Design review of the part shown in the three views and the two pictorial views. Dimensions are in mm from the part's minimum x, y and z. Coordinates: 2 decimals unless noted, no trailing zeros. Loops run counter-clockwise (first coordinate to the right, second up) from the corner with the lowest first, then second, coordinate; pieces in that order, holes last. Notation, with made-up numbers: M 79,-28 L 98,-28 A26 cw 98,-11 Z; hole C 76,-8.5 d1. An arc over 180 degrees is marked long. Put each result on its own line as item: value. Start each with the question number.
(1) Take a section at B-B, the plane y = 2.35. Give the boundary of the cut face in (x, z), then the cut area to 3 significant figures.
(2) Take a section at A-A, the plane z = 14. Give the boundary of the cut face in (x, y), then the cut area to 3 significant figures.
(3) Clearance check with flat-ended pins moving along their axes: pin 1 (1.2 mm diameter, centred on x = 9, z = 29.5, fed in from -Y); pin 2 (3 mm diameter, centred on y = 2, z = 54, fed in from -X); pin 3 (1.2 mm diameter, centred on y = 3, z = 60.5, fed in from +X). State where each tip first meets the part, or that it passes through.
(4) For probe 1 along X at (y, z) = (3.15, 37); probe 2 along Y at (x, z) = (2.5, 58.5), list the stretches that pass through material, from the lowest coordinate up. Write a range as [from, to].
(5) Take a section at C-C, the plane x = 1.5. Give the boundary of the cut face in (y, z).
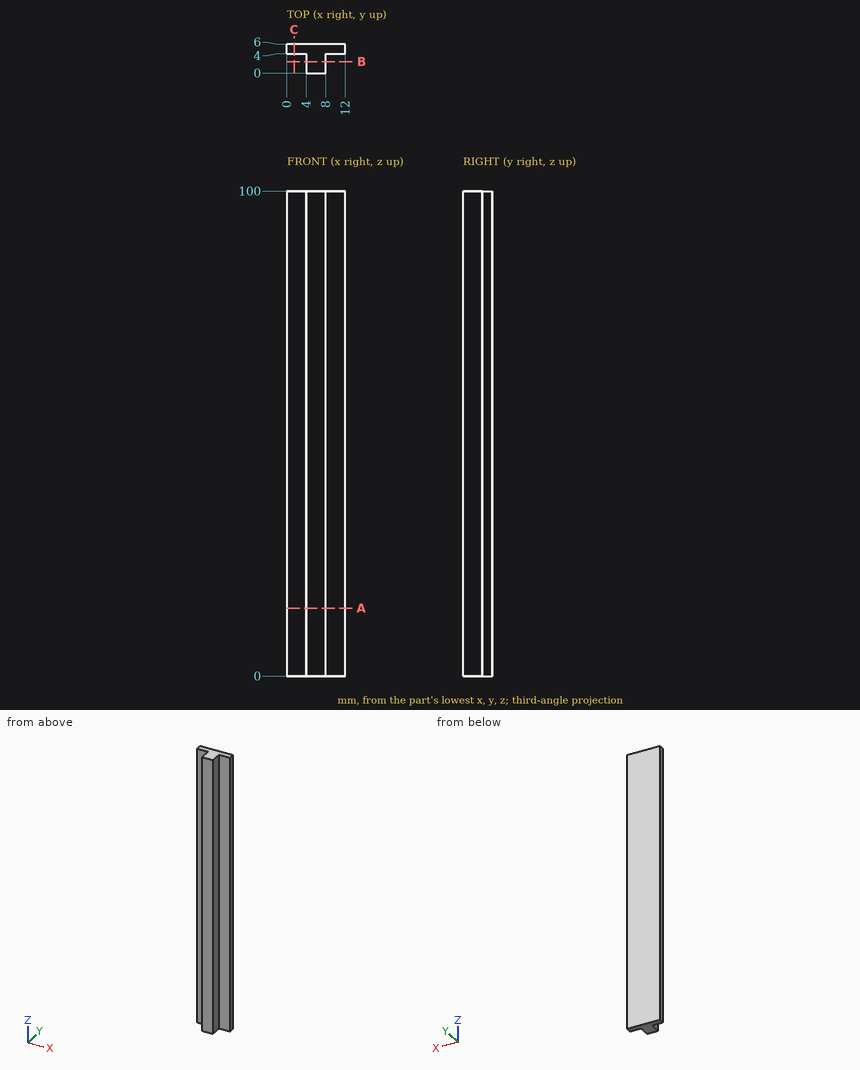
Computed values:
1. outline: M 4,0 L 8,0 L 8,100 L 4,100 Z
1. area: 400 mm^2
2. outline: M 0,4 L 4,4 L 4,0 L 8,0 L 8,4 L 12,4 L 12,6 L 0,6 Z
2. area: 40.0 mm^2
3. pin 1: stops at y = 4
3. pin 2: stops at x = 4
3. pin 3: stops at x = 8
4. probe 1: x = [4, 8]
4. probe 2: y = [4, 6]
5. outline: M 4,0 L 6,0 L 6,100 L 4,100 Z
